Source: three-view drawing plus pictorial views. Frame: mm from the lowest corner of the part. Coordinates: 2 decimals unless noted, no trailing zeros. Write each loop counter-clockwise with the first axis right and the second up, starting at its lowest first coordinate (ties: lowest second). Pieces come first, ordered by that corner, then holes. Notation, with made-up numbers: (45, 43.25) - (73, 43.25) arc R9 cw to (73, 58.25) - close; hole circle Ø4 at (-34.75, 64). An arc over 180 degrees is marked (long way). One line per item, written item: value.
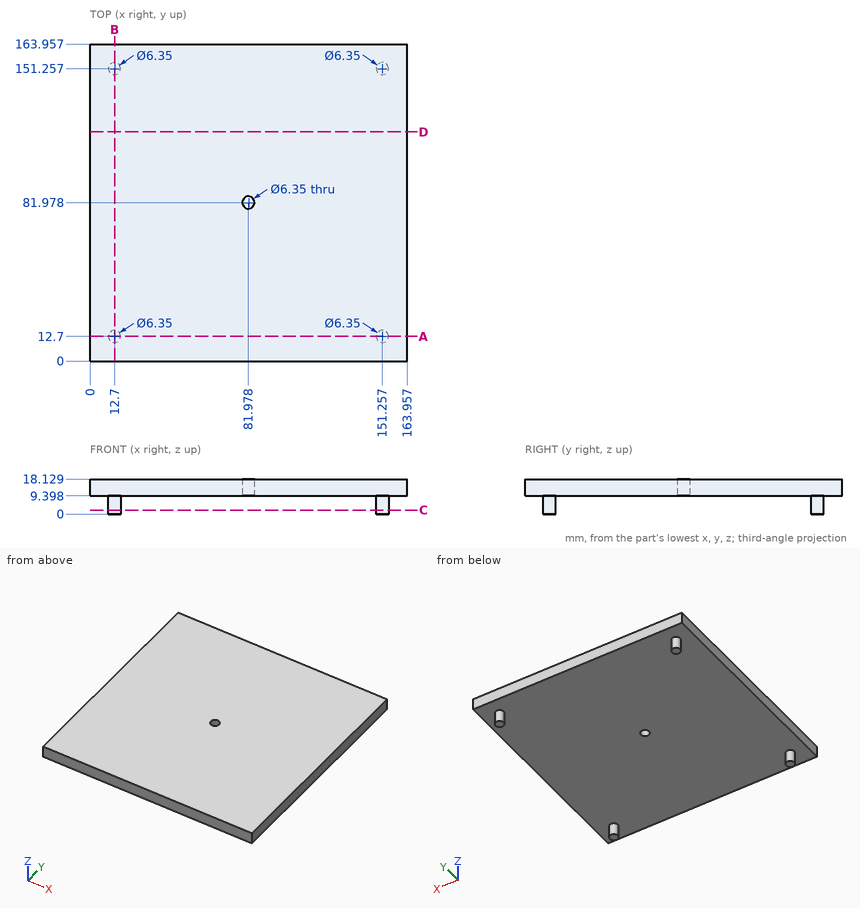
1) Section query D-D on y = 118.5. Output: boundary loops of the cut face in (x, z).
Values found:
outline: (0, 9.4) - (163.96, 9.4) - (163.96, 18.13) - (0, 18.13) - close
2) Contact query for flat-ended pins moving along their axis: P1, Ø3, axis at x = 125.5, y = 46.5, coming from the -Z side; P2, Ø6, axis at x = 24.5, z = 8.5, coming from the +Y side. Output: stop coordinate, or through.
Values found:
P1: z = 9.4
P2: y = 163.96
3) Section query A-A on y = 12.7. Output: boundary loops of the cut face in (x, z) (1 decimal).
Values found:
outline: (0, 9.4) - (9.5, 9.4) - (9.5, 0) - (15.9, 0) - (15.9, 9.4) - (148.1, 9.4) - (148.1, 0) - (154.4, 0) - (154.4, 9.4) - (164, 9.4) - (164, 18.1) - (0, 18.1) - close
4) Section query C-C on z = 2. State how many separate pieces and enclosed holes the cut face has, then the cut area to 3 significant figures.
Values found:
separate pieces: 4
enclosed holes: 0
area: 127 mm2
5) Material intervals for line 1 (Y direction, x = 151, z = 4.5) (1 decimal); line 2 (Z direction, x = 119, y = 18.5); line 3 (Y direction, x = 79.5, z = 15) (1 decimal), sorted ascending.
Values found:
line 1: 9.5 to 15.9, 148.1 to 154.4
line 2: 9.4 to 18.13
line 3: 0 to 80, 84 to 164
